Design review of the part shown in the three views and the two pictorial views. Dimensions are in mm from the part's minimum x, y and z. A direction names the side the tool comes from. Coordinates: 2 decimals unless noted, no trailing zeros. Write each loop counter-clockwise with the first axis right and the second up, starting at its lowest first coordinate (ties: lowest second). Pieces come first, ordered by that corner, then holes. Notation, with made-up numbers: (-3, 11) -> (34, 11) arc R21 cw to (34, 33) -> close; hole circle Ø6 at (45.5, 6.5). An arc over 180 degrees is marked (long way). Write each question's results on one line, items separated by ' | '.
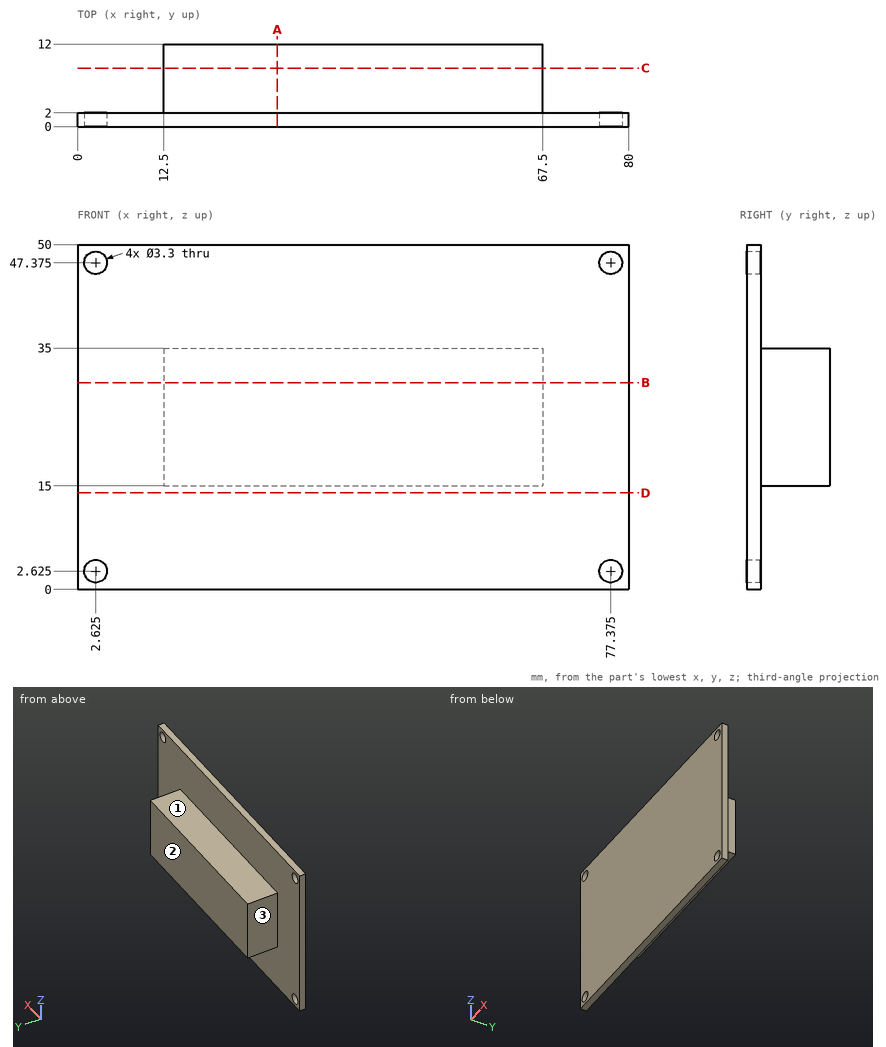
Q1. Machinability: for the marked faces 1, 2 and 3, which of the approach directions +Z, -Z, +X, -X, +Y, -Y give a long, thin tool a straight path to every point of the face, cutting with its end or side? Answer none if there is none.
Solution:
face 1: +Z, +X, -X, +Y | face 2: +Z, -Z, +X, -X, +Y | face 3: +Z, -Z, -X, +Y
Q2. Add section A-A (x = 29). Write out the cut boundary in (y, z), plus the area to 3 significant figures.
Solution:
outline: (0, 0) -> (2, 0) -> (2, 15) -> (12, 15) -> (12, 35) -> (2, 35) -> (2, 50) -> (0, 50) -> close | area: 300 mm²
Q3. Clearance check with flat-ended pins moving along their axes: P1, Ø5, axis at x = 41, y = 7.5, coming from the -Z side; P2, Ø4, axis at x = 77.375, z = 2.625, coming from the +Y side; P3, Ø3, axis at y = 6, z = 22, coming from the +X side; P4, Ø3, axis at x = 77.375, z = 47.375, coming from the -Y side. State where each tip first meets the part, or that it passes through.
Solution:
P1: z = 15 | P2: y = 2 | P3: x = 67.5 | P4: through
Q4. Add section D-D (z = 14). Write out the cut boundary in (x, y).
Solution:
outline: (0, 0) -> (80, 0) -> (80, 2) -> (0, 2) -> close
Q5. Add section C-C (y = 8.5). Write out the cut boundary in (x, z), plus the area to 3 significant figures.
Solution:
outline: (12.5, 15) -> (67.5, 15) -> (67.5, 35) -> (12.5, 35) -> close | area: 1,100 mm²
Q6. For line 1 (Y direction, x = 60.5, z = 7.5); line 2 (X direction, y = 7, z = 22); line 3 (Z direction, x = 38, y = 10), list the stretches that pass through material, from the lowest coordinate up. Write a range as from..to.
Solution:
line 1: 0..2 | line 2: 12.5..67.5 | line 3: 15..35
Q7. Add section B-B (z = 30). Write out the cut boundary in (x, y).
Solution:
outline: (0, 0) -> (80, 0) -> (80, 2) -> (67.5, 2) -> (67.5, 12) -> (12.5, 12) -> (12.5, 2) -> (0, 2) -> close
